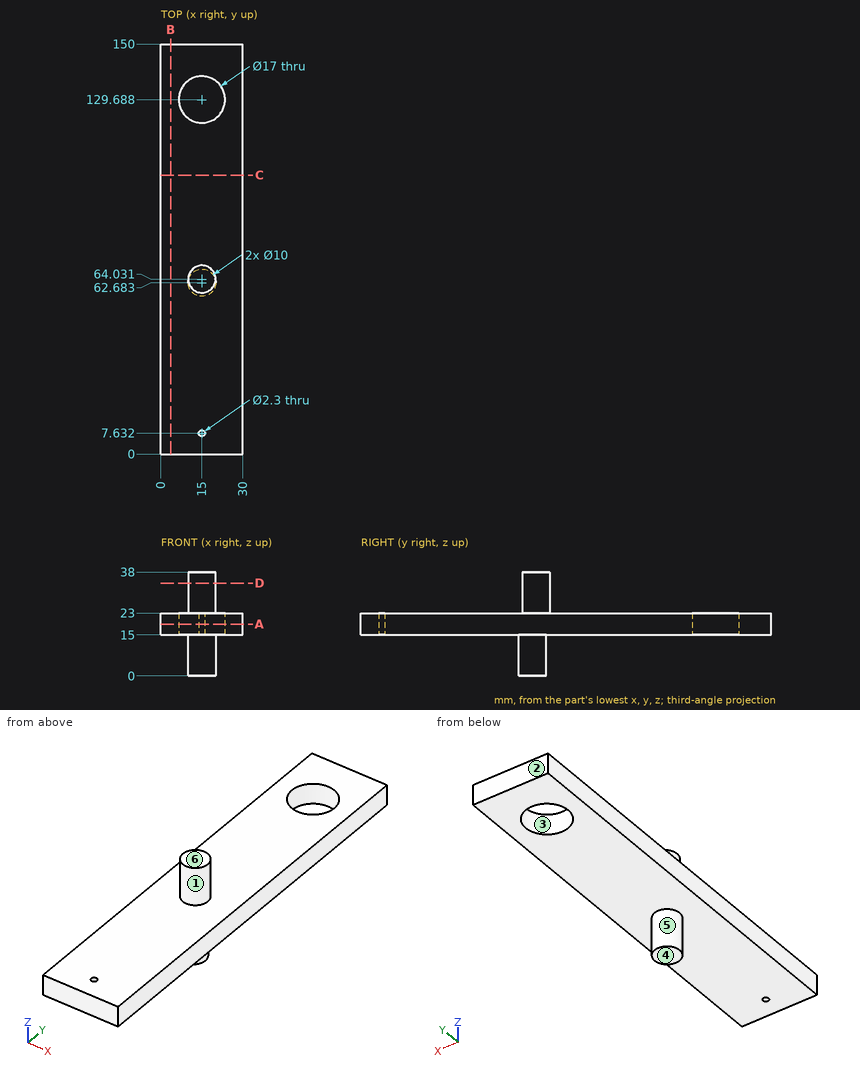
The figure shows three views and two pictorial views of one solid part (mm, origin at its lowest corner). Answer the questions. A direction names the side the tool comes from. Give positions to 0.01 mm unless a question says otherwise; leave off trailing zeros. Write each loop counter-clockwise with the first axis right and the second up, starting at its lowest first coordinate (ties: lowest second). Pieces come first, ordered by that corner, then holes. Notation, with made-up numbers: (12, 42.25) -> (40, 42.25) arc R12 cw to (40, 57.25) -> close; hole circle Ø2 at (79.25, -21.5). An arc over 180 degrees is marked (long way). Write each question's results on one line, items separated by ' | '.
1. Find section C-C on y = 102. Determine the outline of the cut face in (x, z), and give its area (3 significant figures).
Data:
outline: (0, 15) -> (30, 15) -> (30, 23) -> (0, 23) -> close | area: 240 mm^2
2. Straight lines are drawn through the part: L1, parallel to Y at x = 15, z = 19.25; L2, parallel to Z at x = 15, y = 43.5; L3, parallel to Y at x = 20.75, z = 17. For each, find the intervals that lie inside material, in ascending order.
Data:
L1: 0 to 6.48, 8.78 to 121.19, 138.19 to 150 | L2: 15 to 23 | L3: 0 to 123.43, 135.95 to 150
3. A tool of negligible diameter and unlimited length cuts with its end or side. For the marked faces 5 and 6, from which of +Z, -Z, +X, -X, +Y, -Y can it reach the whole face along a straight path? Write none if from no direction.
Data:
face 5: -Z | face 6: +Z, +X, -X, +Y, -Y
4. Each of these flat-tipped pins is pushed along its axis until it touches: pin 1 Ø1 at (x, z) = (15, 24.5) entering from +Y; pin 2 Ø3 at (x, z) = (15, 6) entering from -Y; pin 3 Ø5 at (x, y) = (24, 41) entering from +Z. Where does it stop, or does it pass through?
Data:
pin 1: y = 69.03 | pin 2: y = 57.68 | pin 3: z = 23
5. Find section D-D on z = 34. Determine the outline of the cut face in (x, y).
Data:
outline: circle Ø10 at (15, 64.03)
6. Determine the mould class of the marked faces 1, 2, 3 and 4 for opening direction Y: +Y half, -Y half, draft (parallel to the pull), parting line (faces both ways), or undercut.
Data:
face 1: parting line | face 2: +Y half | face 3: undercut | face 4: draft
7. Find section A-A on z = 19. Determine the outline of the cut face in (x, y).
Data:
outline: (0, 0) -> (30, 0) -> (30, 150) -> (0, 150) -> close; hole circle Ø17 at (15, 129.69); hole circle Ø2.3 at (15, 7.63)
8. Find section B-B on x = 3.5. Determine the outline of the cut face in (y, z), and give its area (3 significant figures).
Data:
outline: (0, 15) -> (150, 15) -> (150, 23) -> (0, 23) -> close | area: 1,200 mm^2
